Autodesk Inventor part; units mm, degrees
ref_plane "YZ Plane" through (0, 0, 0) normal (1, 0, 0) x (0, 1, 0)
ref_plane "XZ Plane" through (0, 0, 0) normal (0, 1, 0) x (-1, 0, 0)
ref_plane "XY Plane" through (0, 0, 0) normal (0, 0, 1) x (1, 0, 0)
sketch "Sketch1" plane through (0, 0, 0) normal (0, 0, 1) x (1, 0, 0)
  line L0 (-6.3366, 6.9163) -> (21.6034, 6.9163)
  line L1 (21.6034, 6.9163) -> (21.6034, -8.3237)
  line L2 (21.6034, -8.3237) -> (-6.3366, -8.3237)
  line L3 (-6.3366, -8.3237) -> (-6.3366, 6.9163)
  point P0 (0, 0)
  dimension "d0" = 27.94
  dimension "d1" = 15.24
extrude "Extrusion1" add sketch "Sketch1" along normal blind 7.62
sketch "Sketch2" plane through (0, 0, 7.62) normal (0, 0, 1) x (1, 0, 0)
  line L0 (-6.3366, 6.9163) -> (-6.3366, -8.3237)
  line L1 (21.6034, -8.3237) -> (21.6034, 6.9163)
  line L2 (21.6034, 1.3937) -> (21.6034, 3.8067)
  line L3 (-6.3366, 3.8067) -> (-6.3366, 1.3937)
  line L4 (21.6034, 6.9163) -> (-6.3366, 6.9163)
  line L5 (-6.3366, -8.3237) -> (21.6034, -8.3237)
  line L6 (0.9631, 3.8067) -> (-0.2406, 3.8067)
  line L7 (-0.2406, 1.3937) -> (0.9631, 1.3937)
  line L8 (-0.2406, 1.3937) -> (-0.2406, 3.8067)
  line L9 (-0.2406, 1.3937) -> (3.0821, 1.3937)
  line L10 (3.0821, 1.3937) -> (3.0821, 3.8067)
  line L11 (3.0821, 3.8067) -> (-0.2406, 3.8067)
  line L12 (-0.2406, 3.8067) -> (-0.2406, 1.3937)
  line L13 (14.3038, 3.8067) -> (15.5074, 3.8067)
  line L14 (15.5074, 1.3937) -> (14.3038, 1.3937)
  line L15 (15.5074, 1.3937) -> (15.5074, 3.8067)
  line L16 (15.5074, 1.3937) -> (12.1847, 1.3937)
  line L17 (12.1847, 1.3937) -> (12.1847, 3.8067)
  line L18 (12.1847, 3.8067) -> (15.5074, 3.8067)
  line L19 (15.5074, 3.8067) -> (15.5074, 1.3937)
  line L20 (-6.3366, -0.7037) -> (21.6034, -0.7037)
  line L21 (-6.3366, 3.8067) -> (21.6034, 3.8067)
  line L22 (21.6034, 3.8067) -> (21.6034, 1.3937)
  line L23 (21.6034, 1.3937) -> (-6.3366, 1.3937)
  line L24 (-6.3366, 1.3937) -> (-6.3366, 3.8067)
  point P0 (0, 0)
  point P1 (-0.2406, 2.6002)
  point P2 (15.2669, 1.0813)
  point P3 (15.5074, 2.6002)
  point P4 (15.5074, 1.3937)
  point P5 (21.6034, 3.8067)
  point P6 (15.5074, 3.8067)
  point P7 (-0.2406, 1.3937)
  point P8 (-0.2406, 3.8067)
  point P9 (-6.3366, 3.8067)
  point P10 (3.0821, 1.3937)
  point P11 (12.1847, 1.3937)
  point P12 (12.1847, 3.8067)
  point P13 (3.0821, 3.8067)
  dimension "d6" = 6.096
extrude "Extrusion2" add sketch "Sketch2" along normal blind 8.7376 contours L6 L11 L10 L9 L7 L8 | L15 L14 L16 L17 L18 L13
sketch "Sketch3" plane through (-0.2406, 3.8067, 7.62) normal (0, 1, 0) x (1, 0, 0)
  line L0 (3.3227, -8.7376) -> (0, -8.7376)
  line L1 (-6.096, 7.62) -> (21.844, 7.62)
  line L2 (3.3227, -11.3552) -> (3.3227, -8.7376)
  line L3 (12.4253, -11.3552) -> (12.4253, -8.7376)
  line L4 (17.2091, -8.255) -> (17.2091, -15.2732)
  line L5 (17.2091, -15.2732) -> (14.9854, -19.057)
  line L6 (14.9854, -19.057) -> (12.4253, -19.057)
  line L7 (12.4253, -19.057) -> (12.4253, -8.7376)
  line L8 (7.874, 7.62) -> (7.874, -24.8322)
  line L9 (3.3227, -11.3552) -> (3.3227, -8.7376)
  line L10 (-1.4611, -8.255) -> (-1.4611, -15.2732)
  line L11 (-1.4611, -15.2732) -> (0.7626, -19.057)
  line L12 (0.7626, -19.057) -> (3.3227, -19.057)
  line L13 (3.3227, -19.057) -> (3.3227, -8.7376)
  line L14 (17.2091, -8.255) -> (12.4253, -8.255)
  line L15 (12.4253, 0) -> (12.4253, -8.7376)
  line L16 (12.4253, -8.255) -> (12.4253, -8.7376)
  line L17 (-1.4611, -8.255) -> (3.3227, -8.255)
  line L18 (3.3227, 0) -> (3.3227, -8.7376)
  line L19 (3.3227, -8.255) -> (3.3227, -8.7376)
  point P0 (0.2406, 7.62)
extrude "Extrusion4" add sketch "Sketch2" along normal blind 25.4 contours L6 L11 L10 L9 L7 L8 | L15 L14 L16 L17 L18 L13
sketch "Sketch4" plane through (-6.3366, 6.9163, 0) normal (0, 1, 0) x (1, 0, 0)
  point P0 (6.3366, 0)
sketch "Sketch5" plane through (0, 0, 7.62) normal (0, 0, 1) x (1, 0, 0)
  line L0 (21.6034, 6.9163) -> (-6.3366, 6.9163)
  line L1 (-6.3366, 15.6735) -> (21.6034, 15.6735)
  line L2 (21.6034, 15.6735) -> (21.6034, 6.9163)
  line L3 (21.6034, 6.9163) -> (-6.3366, 6.9163)
  line L4 (-6.3366, 6.9163) -> (-6.3366, 15.6735)
  point P0 (0, 0)
extrude "Extrusion5" add sketch "Sketch5" along normal blind 17.145 and the other way blind 7.62
extrude "Extrusion6" cut sketch "Sketch2" against normal blind 25.4 contours L20 L1 L5 L0
extrude "Extrusion7" add sketch "Sketch2" along normal blind 4.7625 contours L21 L8 L23 L0 | L1 L23 L15 L21 | L21 L17 L23 L10
extrude "Extrusion8" add sketch "Sketch3" against normal up to surface (2.413 mm away)
sketch "Sketch6" plane through (-6.3366, 1.3937, 7.62) normal (0, -1, 0) x (1, 0, 0)
  line L0 (27.94, 0) -> (27.94, 4.7625)
  line L1 (21.844, 4.7625) -> (21.844, 8.255)
  line L2 (27.94, 0) -> (21.844, 0)
  line L3 (21.844, 0) -> (21.844, 4.7625)
  line L4 (21.844, 4.7625) -> (27.94, 4.7625)
  line L5 (27.94, 4.7625) -> (27.94, 0)
  line L6 (18.5213, 4.7625) -> (18.5213, 25.4)
  line L7 (18.5213, 4.7625) -> (9.4187, 4.7625)
  line L8 (9.4187, 4.7625) -> (9.4187, 0)
  line L9 (9.4187, 0) -> (18.5213, 0)
  line L10 (18.5213, 0) -> (18.5213, 4.7625)
  line L11 (6.096, 4.7625) -> (6.096, 8.255)
  line L12 (0, 0) -> (0, 4.7625)
  line L13 (6.096, 4.7625) -> (0, 4.7625)
  line L14 (0, 4.7625) -> (0, 0)
  line L15 (0, 0) -> (6.096, 0)
  line L16 (6.096, 0) -> (6.096, 4.7625)
  point P0 (6.3366, -7.62)
  point P1 (21.844, 8.7376)
  point P2 (18.5213, 19.057)
  point P3 (6.096, 8.7376)
extrude "Extrusion9" cut sketch "Sketch6" against normal up to surface (5.5227 mm away)
sketch "Sketch7" plane through (12.1847, 1.3937, 7.62) normal (0, -1, 0) x (1, 0, 0)
  line L0 (3.3227, 17.7594) -> (4.7838, 15.2732)
  line L1 (3.3227, 17.7594) -> (2.3659, 19.3874)
  line L2 (2.3659, 19.3874) -> (2.3659, 25.4)
  line L3 (3.3227, 25.4) -> (0, 25.4)
  line L4 (3.3227, 17.7594) -> (3.3227, 25.4)
  line L5 (2.3659, 25.4) -> (3.3227, 25.4)
  line L6 (3.3227, 25.4) -> (3.3227, 17.7594)
  line L7 (-18.5213, -7.62) -> (9.4187, -7.62)
  line L8 (-12.4253, 17.7594) -> (-11.4685, 19.3874)
  line L9 (-11.4685, 19.3874) -> (-11.4685, 25.4)
  line L10 (-12.4253, 17.7594) -> (-12.4253, 25.4)
  line L11 (-11.4685, 25.4) -> (-12.4253, 25.4)
  line L12 (-12.4253, 25.4) -> (-12.4253, 17.7594)
  line L13 (-12.4253, 8.7376) -> (-13.8865, 8.255)
  line L14 (-9.1825, 8.7376) -> (-9.1026, 8.7376)
  line L15 (-9.1026, 0) -> (-9.1026, 25.4)
  line L16 (-10.6842, 5.3569) -> (-10.764, 0)
  line L17 (-9.1026, 0) -> (-12.4253, 0)
  line L18 (-9.1026, 0) -> (-9.1026, 8.7376)
  line L19 (-10.764, 0) -> (-9.1026, 0)
  line L20 (9.4187, -7.62) -> (-18.5213, -7.62)
  line L21 (-18.5213, 17.145) -> (9.4187, 17.145)
  line L22 (1.5816, 5.3569) -> (1.6613, 0)
  line L23 (1.6613, 0) -> (0, 0)
  line L24 (0, 0) -> (0, 8.7376)
  line L25 (-4.5513, -7.62) -> (-4.5513, 0)
  line L26 (-4.5513, 11.274) -> (-4.5513, 11.3382)
  line L27 (-9.1026, 8.7376) -> (-10.6842, 5.3569)
  line L28 (0, 8.7376) -> (1.5816, 5.3569)
  point P0 (-12.1847, -7.62)
extrude "Extrusion10" cut sketch "Sketch7" against normal up to surface (5.5227 mm away)
fillet "Fillet1" radius 3.175 4 edges at (0.7162, 2.6002, 33.02) (14.5507, 2.6002, 33.02) (16.9686, 2.6002, 22.8932) (-1.7017, 2.6002, 22.8932)
sketch "Sketch8" plane through (-0.2406, 1.3937, 7.62) normal (0, -1, 0) x (1, 0, 0)
  arc A0 (-1.0234, 16.018) -> (-1.4611, 14.4093) centre (1.7139, 14.4093) ccw
  line L0 (-1.4611, 8.255) -> (-1.4611, 14.4093)
  line L1 (0, 0) -> (0, 8.255)
  line L2 (1.6613, 0) -> (0, 0)
  line L3 (1.6613, 0) -> (1.7411, 5.3569)
  line L4 (1.7411, 5.3569) -> (3.3227, 8.7376)
  line L5 (3.3227, 8.7376) -> (3.3227, 25.4)
  arc A1 (3.3227, 25.4) -> (0.9568, 22.3298) centre (4.1318, 22.3298) ccw
  line L6 (0.9568, 22.3298) -> (0.9568, 19.3874)
  line L7 (0.9568, 19.3874) -> (-1.0234, 16.018)
  arc A2 (17.2091, 14.4093) -> (16.7714, 16.018) centre (14.0341, 14.4093) ccw
  line L8 (16.7714, 16.018) -> (14.7912, 19.3874)
  line L9 (14.7912, 19.3874) -> (14.7912, 22.3298)
  arc A3 (14.7912, 22.3298) -> (12.4253, 25.4) centre (11.6162, 22.3298) ccw
  line L10 (12.4253, 8.7376) -> (12.4253, 25.4)
  line L11 (12.4253, 8.7376) -> (14.0069, 5.3569)
  line L12 (14.0069, 5.3569) -> (14.0867, 0)
  line L13 (15.748, 0) -> (14.0867, 0)
  line L14 (15.748, 0) -> (15.748, 8.255)
  line L15 (17.2091, 14.4093) -> (17.2091, 8.255)
  line L16 (17.2091, 8.255) -> (15.748, 8.255)
  line L17 (0, 8.255) -> (-1.4611, 8.255)
  point P0 (0.2406, -7.62)
extrude "Extrusion11" add sketch "Sketch8" against normal blind 3.81
sketch "Sketch9" plane through (0, 0, 7.62) normal (0, 0, 1) x (1, 0, 0)
  line L0 (9.6447, 1.3599) -> (5.6221, 1.3599)
  line L1 (5.6221, 1.3599) -> (5.6221, 5.1699)
  line L2 (5.6221, 5.1699) -> (9.6447, 5.1699)
  line L3 (9.6447, 5.1699) -> (9.6447, 1.3599)
  line L4 (12.1847, 1.3937) -> (12.1847, 5.2037)
  line L5 (3.0821, 1.3937) -> (3.0821, 5.2037)
  line L6 (1.4208, 1.3937) -> (1.4208, 5.2037)
  point P0 (0, 0)
  dimension "d30" = 2.54
  dimension "d31" = 2.54
extrude "Extrusion12" add sketch "Sketch9" along normal blind 18.0975
properties part number "Attachment4"
The model under review builds one solid part; all positions refer to its coordinate system, in mm. A direction names the side the tool comes from. Round coordinates to 2 decimals unless told otherwise and drop trailing zeros. Loops run counter-clockwise (first coordinate to the right, second up) from the corner with the lowest first, then second, coordinate; pieces in that order, holes last. Notation, with made-up numbers: M -20,56 L 17,56 A18 ccw 17,66 Z; hole C 2.5,-3 d3. An arc over 180 degrees is marked long. Write item = value, one per line.
Item 1: Take a section at C-C on x = 7. Write out the cut boundary in (y, z) (1 decimal).
Return value:
outline = M -0.7,0 L 15.7,0 L 15.7,24.8 L 6.9,24.8 L 6.9,7.6 L 5.2,7.6 L 5.2,25.7 L 1.4,25.7 L 1.4,7.6 L -0.7,7.6 Z
Item 2: Take a section at A-A on x = 11.75. Write out the cut boundary in (y, z) (1 decimal).
Return value:
outline = M -0.7,0 L 15.7,0 L 15.7,24.8 L 6.9,24.8 L 6.9,7.6 L -0.7,7.6 Z
Item 3: Take a section at D-D on y = 12.25. Write out the cut boundary in (x, z) (3 decimals), then the cut area to 3 significant figures.
Return value:
outline = M -6.337,0 L 21.603,0 L 21.603,24.765 L -6.337,24.765 Z
area = 692 mm2
Item 4: For line 1 (Y direction, x = 1.5, z = 14); line 2 (X direction, y = 4, z = 30); line 3 (Z direction, x = 16, y = 12.75) (3 decimals), list the stretches that pass through material, from the lowest coordinate up. Write a range as [from, to].
Return value:
line_1 = [1.39, 5.2], [6.92, 15.67]
line_2 = [0.72, 3.08], [12.18, 14.55]
line_3 = [0, 24.765]
Item 5: Insertion check: P1, Ø1.1, axis at y = 3.5, z = 27.5, coming from the +X side; P2, Ø2.5, axis at x = 8.5, z = 9.5, coming from the -Y side; P3, Ø4, axis at y = 4, z = 10.5, coming from the +X side. Each pin has a flat end and moves straight along its axis. Give the tip position at first contact, or say it passes through.
Return value:
P1 = 14.58
P2 = 1.36
P3 = 15.51
Item 6: The part is to be moulded in two halves that separate along X. For faces 5 (the flat face through (0.716, 3, 28)), 6 (the flat face through (7, 8, 0)), 7 (the flat face through (8, 3, 25.718)), say which applies: released by +X, released by -X, zero draft, split by the parting line, or undercut.
Return value:
face_5 = released by -X
face_6 = zero draft
face_7 = undercut
Item 7: Machinability: for faces 1 (the flat face through (8, 1.36, 17)), 2 (the flat face through (15.507, 3, 12)), 3 (the flat face through (-1.702, 3, 19)), 4 (the flat face through (14, 5.204, 20)), which of the approach directions +Z, -Z, +X, -X, +Y, -Y give a long, thin tool a straight path to every point of the face, cutting with its end or side? Answer none if there is none.
Return value:
face_1 = +Z, +X, -X, -Y
face_2 = +X, -Y
face_3 = +Z, -X, -Y
face_4 = +Z, +X, -X
